Autodesk Inventor part; units mm, degrees
ref_plane "YZ Plane" through (0, 0, 0) normal (1, 0, 0) x (0, 1, 0)
ref_plane "XZ Plane" through (0, 0, 0) normal (0, 1, 0) x (-1, 0, 0)
ref_plane "XY Plane" through (0, 0, 0) normal (0, 0, 1) x (1, 0, 0)
sketch "Sketch1" plane through (0, 0, 0) normal (1, 0, 0) x (0, 1, 0)
  line L0 (0, 12.6765) -> (0, -12.6765)
  line L1 (0, 0) -> (2, 0)
  line L2 (2, 0) -> (2, 10)
  line L3 (2, 10) -> (5.25, 10)
  line L4 (5.25, 10) -> (5.25, 7)
  line L5 (5.25, 7) -> (4, 7)
  line L6 (4, 7) -> (4, -3)
  line L7 (4, -3) -> (3.19, -3)
  line L8 (3.19, -3) -> (3.19, -8)
  line L9 (3.19, -8) -> (2.75, -8)
  line L10 (2.75, -8) -> (2.75, -11.3)
  line L11 (2.75, -11.3) -> (0, -11.3)
  line L12 (0, -11.3) -> (0, 0)
  line L13 (2.75, -18.5) -> (0, -18.5) construction
  point P0 (2, 5)
  dimension "d0" = 4
  dimension "d1" = 3
  dimension "d2" = 10
  dimension "d3" = 10.5
  dimension "d4" = 8
  dimension "d5" = 6.38
  dimension "d6" = 5.5
  dimension "d7" = 28.5
  dimension "d8" = 10.5
  dimension "d9" = 21.3
  dimension "d10" = 13
revolve "Revolution1" add sketch "Sketch1" angle 360 about axis through (0, 0, 12.6765) along (0, 0, -1)
properties part number "A-2.103-B"
Input: part model. Units: mm. Frame: model coordinates. A direction names the side the tool comes from. Coordinates: 2 decimals unless noted, no trailing zeros. Loops run counter-clockwise (first coordinate to the right, second up) from the corner with the lowest first, then second, coordinate; pieces in that order, holes last. Notation, with made-up numbers: (29.5, 13) -> (78.5, 13) arc R11 ccw to (78.5, 29) -> close; hole circle Ø2 at (0, 83.5). An arc over 180 degrees is marked (long way). Write item = value, one per line. Start each with the question number.
Item 1: First-contact query: P1, Ø5, axis at y = -4, z = 6.5, coming from the +X side; P2, Ø6, axis at y = -2, z = 5.5, coming from the -X side; P3, Ø1.5, axis at y = 4, z = 5.5, coming from the -X side; P4, Ø1.5, axis at y = 1.5, z = -0.5, coming from the +X side. Flat tips, straight axial feed; report the tip coordinate or a pass-through.
Item 2: Cut plane B-B, the plane z = 8.5. Return loops of the section in (x, y).
Item 3: Cut plane D-D, the plane z = -2.25. Return loops of the section in (x, y), plus the area to 3 significant figures.
Item 4: Cut plane A-A, the plane x = 0. Return loops of the section in (y, z).
Item 5: Mould query, pull axis Y, two halves, no side actions, for faces 1 (the face through (-2, -4, 7)), 2 (the face through (0, 0, 0)), 3 (the face through (1.6, 5, 8.5)), 4 (the face through (2, 0, 5)). Classes: pulls with the +Y half, pulls with the -Y half, needs draft (parallel to the pull), parting line crosses it, or undercut.
Item 6: Material intervals for line 1 (X direction, y = 0, z = 4); line 2 (X direction, y = 0, z = 7.75); line 3 (Z direction, x = -0.75, y = -1.5), sorted ascending.
Item 7: Reachability of faces 5 (the face through (-2.685, -0.596, -9.673)), 6 (the face through (0.1, 2.3, 10)) from +Z, -Z, +X, -X, +Y, -Y: full face, straight path, thin tool, end or side. Return the list, or none.
Ans:
q1.P1 = 5.02
q1.P2 = -5.25
q1.P3 = -2.33
q1.P4 = 3.93
q2.outline = circle Ø10.5 at (0, 0); hole circle Ø4 at (0, 0)
q3.outline = circle Ø8 at (0, 0)
q3.area = 50.3 mm²
q4.outline = (-5.25, 7) -> (-4, 7) -> (-4, -3) -> (-3.19, -3) -> (-3.19, -8) -> (-2.75, -8) -> (-2.75, -11.3) -> (2.75, -11.3) -> (2.75, -8) -> (3.19, -8) -> (3.19, -3) -> (4, -3) -> (4, 7) -> (5.25, 7) -> (5.25, 10) -> (2, 10) -> (2, 0) -> (-2, 0) -> (-2, 10) -> (-5.25, 10) -> close
q5.face_1 = needs draft
q5.face_2 = undercut
q5.face_3 = parting line crosses it
q5.face_4 = undercut
q6.line_1 = -4 to -2, 2 to 4
q6.line_2 = -5.25 to -2, 2 to 5.25
q6.line_3 = -11.3 to 0
q7.face_5 = -Z
q7.face_6 = +Z, +X, -X, +Y, -Y
